Design review of the part built by this model. Coordinates are the model's own, in mm. A direction names the side the tool comes from. Round coordinates to 2 decimals unless told otherwise and drop trailing zeros. Order: outer loops, then holes, each group sorted by start corner. A loop starts at its lowest first (then second) coordinate and runs counter-clockwise, first axis right, second up.
from build123d import *

# Parameters (mm, degrees)
F0_W      = 50.8
F0_H      = 57.15
F1_DEPTH  = 31.75
F3_DEPTH  = 50.8
F4_W      = 12.7
F4_H      = 25.4
F5_DEPTH  = 25.4
F6_W      = 12.7
F6_H      = 12.7
F7_DEPTH  = 25.4
F9_DEPTH  = 25.4
F11_DEPTH = 25.4
F13_DEPTH = 12.7
F14_R     = 6.7335002537
F15_DEPTH = 25.4
F17_DEPTH = 25.4
F18_R     = 1.6140947443
F18_R_2   = 1.6110130755
F19_DEPTH = 25.4


with BuildPart() as f1:
    # F0 (on Front) → F1 (new body)
    with BuildSketch(Plane.XZ):
        with Locations((-43.8855561577, 28.575)):
            Rectangle(F0_W, F0_H)
    extrude(amount=F1_DEPTH)

    # F2 (on face) → F3 (cut)
    with BuildSketch(Plane(origin=(-69.2855561577, 0, 0), x_dir=(0, -1, 0), z_dir=(-1, 0, 0))):
        Polygon((12.7, 6.35), (31.75, 6.35), (31.75, 57.15), (25.4, 57.15), (25.4, 31.75), (12.7, 31.75), align=None)
    extrude(amount=-F3_DEPTH, mode=Mode.SUBTRACT)

    # F4 (on face) → F5 (cut)
    with BuildSketch(Plane.XZ.offset(25.4)):
        with Locations((-24.8355561577, 44.45)):
            Rectangle(F4_W, F4_H)
        with Locations((-62.9355561577, 44.45)):
            Rectangle(F4_W, F4_H)
    extrude(amount=-F5_DEPTH, mode=Mode.SUBTRACT)

    # F6 (on face) → F7 (cut)
    with BuildSketch(Plane.XZ.offset(12.7)):
        with Locations((-62.9355561577, 25.4)):
            Rectangle(F6_W, F6_H)
        with Locations((-24.8355561577, 25.4)):
            Rectangle(F6_W, F6_H)
    extrude(amount=-F7_DEPTH, mode=Mode.SUBTRACT)

    # F8 (on face) → F9 (cut)
    with BuildSketch(Plane.XZ.offset(12.7)):
        with BuildLine():
            Line((-69.2855561577, 19.05), (-69.2855561577, 6.35))
            ThreePointArc((-69.2855561577, 6.35), (-60.3053000366, 10.0697438789), (-56.5855561577, 19.05))
            Line((-56.5855561577, 19.05), (-69.2855561577, 19.05))
        make_face()
        with BuildLine():
            ThreePointArc((-31.1855561577, 19.05), (-27.4658122788, 10.0697438789), (-18.4855561577, 6.35))
            Line((-18.4855561577, 6.35), (-18.4855561577, 19.05))
            Line((-18.4855561577, 19.05), (-31.1855561577, 19.05))
        make_face()
    extrude(amount=-F9_DEPTH, mode=Mode.SUBTRACT)

    # F10 (on face) → F11 (cut)
    with BuildSketch(Plane.XZ.offset(25.4)):
        with BuildLine():
            Line((-56.5855561577, 57.15), (-56.5855561577, 44.7837235148))
            ThreePointArc((-56.5855561577, 44.7837235148), (-53.5129172667, 52.9012905804), (-45.9442665885, 57.15))
            Line((-45.9442665885, 57.15), (-56.5855561577, 57.15))
        make_face()
        with BuildLine():
            ThreePointArc((-41.8268457269, 57.15), (-34.2581950488, 52.9012905804), (-31.1855561577, 44.7837235148))
            Line((-31.1855561577, 44.7837235148), (-31.1855561577, 57.15))
            Line((-31.1855561577, 57.15), (-41.8268457269, 57.15))
        make_face()
    extrude(amount=-F11_DEPTH, mode=Mode.SUBTRACT)

    # F12 (on face) → F13 (cut)
    with BuildSketch(Plane.XZ.offset(25.4)):
        with BuildLine():
            ThreePointArc((-31.1855561577, 44.5365372296), (-43.8855561577, 31.9595289981), (-56.5855561577, 44.5365372296))
            Line((-56.5855561577, 44.5365372296), (-56.5855561577, 31.75))
            Line((-56.5855561577, 31.75), (-31.1855561577, 31.75))
            Line((-31.1855561577, 31.75), (-31.1855561577, 44.5365372296))
        make_face()
    extrude(amount=-F13_DEPTH, mode=Mode.SUBTRACT)

    # F14 (on face) → F15 (cut)
    with BuildSketch(Plane.XZ.offset(25.4)):
        with Locations((-43.8855561577, 44.6168617574)):
            Circle(F14_R)
    extrude(amount=-F15_DEPTH, mode=Mode.SUBTRACT)

    # F16 (on face) → F17 (cut)
    with BuildSketch(Plane.XY.offset(6.35)):
        with BuildLine():
            ThreePointArc((-64.719619815, -31.75), (-67.8220929264, -30.0962429481), (-69.2855561577, -26.8995998395))
            Line((-69.2855561577, -26.8995998395), (-69.2855561577, -31.75))
            Line((-69.2855561577, -31.75), (-64.719619815, -31.75))
        make_face()
        with BuildLine():
            Line((-18.4855561577, -31.75), (-18.4855561577, -25.7653463632))
            ThreePointArc((-18.4855561577, -25.7653463632), (-20.2347846396, -29.5237639054), (-23.7318370491, -31.75))
            Line((-23.7318370491, -31.75), (-18.4855561577, -31.75))
        make_face()
    extrude(amount=-F17_DEPTH, mode=Mode.SUBTRACT)

    # F18 (on face) → F19 (cut)
    with BuildSketch(Plane.XY.offset(6.35)):
        with Locations((-63.8238352858, -26.3324731014)):
            Circle(F18_R)
        with Locations((-23.7318370491, -26.3324731014)):
            Circle(F18_R_2)
    extrude(amount=-F19_DEPTH, mode=Mode.SUBTRACT)


solid = f1.part
1) Take a section at B-B on x = -47.5. Give the boundary of the cut face in (y, z), plus the area to 3 significant figures.
Results:
outline: (-31.75, 0) - (0, 0) - (0, 38.94) - (-25.4, 38.94) - (-25.4, 32.48) - (-12.7, 32.48) - (-12.7, 6.35) - (-31.75, 6.35) - close; (-25.4, 50.3) - (0, 50.3) - (0, 56.79) - (-25.4, 56.79) - close
area: 862 mm2
2) Take a section at A-A on y = -17.5. Give the boundary of the cut face in (x, z).
Results:
outline: (-69.29, 0) - (-18.49, 0) - (-18.49, 6.35) - (-69.29, 6.35) - close; (-56.59, 44.54) arc R12.7 ccw to (-31.19, 44.54) - (-31.19, 44.78) arc R12.7 ccw to (-41.83, 57.15) - (-45.94, 57.15) arc R12.7 ccw to (-56.59, 44.78) - close; hole circle Ø13.47 at (-43.89, 44.62)
3) Take a section at D-D on z = 46.5. Give the boundary of the cut face in (x, y), plus the area to 3 significant figures.
Results:
outline: (-56.45, -25.4) - (-50.35, -25.4) - (-50.35, 0) - (-56.45, 0) - close; (-37.42, -25.4) - (-31.32, -25.4) - (-31.32, 0) - (-37.42, 0) - close
area: 310 mm2
4) For faces 1 (the face through (-56.586, -7, 32)), 2 (the face through (-43.608, -19.139, 31.963)), 3 (the face through (-69.286, -13, 3)), 4 (the face through (-38, -25.4, 39)), 5 (the face through (-31.186, -7, 32)), list the 3-axis set-ups (+Z, -Z, +X, -X, +Y, -Y) from which the entire face can be reached by the end or side of a thin tool; tool diameter is ignored.
Results:
face 1: +Z, -X, +Y, -Y
face 2: -Y
face 3: +Z, -Z, -X, +Y, -Y
face 4: +Z, +X, -X, -Y
face 5: +Z, +X, +Y, -Y
5) To check wall thickness, follow line 1 along X through (y, z) = (-4, 30.5); line 2 along Y through (x, z) = (-46, 8.5); line 3 along X through (y, z) = (-10, 44.5). State the ranges of each line that lie inside material, in increasing order.
Results:
line 1: x = -56.59 to -31.19
line 2: y = -12.7 to 0
line 3: x = -56.59 to -50.62, -37.15 to -31.19
6) The part is to be moulded in two halves that separate along Z. For faces 6 (the face through (-49.23, -12.88, 40.52)), 7 (the face through (-44, -22, 6.35)), 8 (the face through (-18.486, -13, 3)), 9 (the face through (-34.34, -12.878, 52.995)), say which applies: released by +Z, released by -Z, zero draft, split by the parting line, or undercut.
Results:
face 6: undercut
face 7: undercut
face 8: zero draft
face 9: released by +Z
7) Take a section at C-C on z = 5.5. Give the boundary of the cut face in (x, y).
Results:
outline: (-69.29, -26.9) arc R5.49 ccw to (-64.72, -31.75) - (-23.73, -31.75) arc R7.39 ccw to (-18.49, -25.77) - (-18.49, 0) - (-69.29, 0) - close; hole circle Ø3.23 at (-63.82, -26.33); hole circle Ø3.22 at (-23.73, -26.33)
8) Clearance check with flat-ended pins moving along their axes: P1, Ø8, axis at x = -53.5, z = 27.5, coming from the -Y side; P2, Ø4, axis at y = -26.5, z = 49.5, coming from the +X side; P3, Ø12.5, axis at y = -15, z = 25.5, coming from the +X side. State where each tip first meets the part, or that it passes through.
Results:
P1: stops at y = -12.7
P2: stops at x = -31.6
P3: stops at x = -31.19
